Model file for the job. Use its own axes, mm. A direction names the side the tool comes from. Coordinates: 2 decimals unless noted, no trailing zeros. Order: outer loops, then holes, each group sorted by start corner. A loop starts at its lowest first (then second) coordinate and runs counter-clockwise, first axis right, second up.
from build123d import *

# Parameters (mm, degrees)
BOSS_EXTRUDE1_DEPTH      = 10
BOSS_EXTRUDE2_DEPTH      = 15
BOSS_EXTRUDE2_DEPTH_BACK = 25
SKETCH2_W                = 13.86324318
SKETCH2_H                = 2.640648634
SKETCH3_R                = 3.15
CUT_EXTRUDE1_DEPTH       = 2.65
BOSS_EXTRUDE3_DEPTH      = 10
SKETCH5_R                = 3.15
CUT_EXTRUDE2_DEPTH       = 10
BOSS_EXTRUDE4_DEPTH      = 15
BOSS_EXTRUDE4_DEPTH_BACK = 25
SKETCH7_W                = 13.86324318
SKETCH7_H                = 33.4262151
CUT_EXTRUDE3_DEPTH       = 15
SKETCH13_W               = 7.942289342
SKETCH13_H               = 13.358433402
SKETCH13_H_2             = 13.079806518
CUT_EXTRUDE4_DEPTH       = 35


with BuildPart() as part:
    # Sketch1 → Boss-Extrude1 (new body)
    with BuildSketch(Plane.XY):
        with BuildLine():
            Line((-102.490463188, 678.270987862), (-97.502783366, 678.270987862))
            ThreePointArc((-97.502783366, 678.270987862), (-96.402724844, 679.006023468), (-96.660835024, 680.30363097))
            Line((-96.660835024, 680.30363097), (-101.554583476, 685.197379422))
            ThreePointArc((-101.554583476, 685.197379422), (-102.523344038, 685.844684534), (-103.666075035, 686.071987862))
            Line((-103.666075035, 686.071987862), (-109.332102168, 686.071987862))
            ThreePointArc((-109.332102168, 686.071987862), (-110.474833165, 685.844684534), (-111.443593727, 685.197379422))
            Line((-111.443593727, 685.197379422), (-116.337342179, 680.30363097))
            ThreePointArc((-116.337342179, 680.30363097), (-116.595452359, 679.006023468), (-115.495393837, 678.270987862))
            Line((-115.495393837, 678.270987862), (-112.290288601, 678.270987862))
            Line((-112.290288601, 678.270987862), (-110.43275253, 678.270987862))
            Line((-110.43275253, 678.270987862), (-110.43275253, 674.001864678))
            Line((-110.43275253, 674.001864678), (-113.469742626, 674.001864678))
            Line((-113.469742626, 674.001864678), (-113.469742626, 640.576503739))
            Line((-113.469742626, 640.576503739), (-113.469742626, 637.935000944))
            Line((-113.469742626, 637.935000944), (-99.606499446, 637.935000944))
            Line((-99.606499446, 637.935000944), (-99.606499446, 674.001864678))
            Line((-99.606499446, 674.001864678), (-102.490463188, 674.001864678))
            Line((-102.490463188, 674.001864678), (-102.490463188, 678.270987862))
        make_face()
    extrude(amount=-BOSS_EXTRUDE1_DEPTH)

    # Sketch2 → Boss-Extrude2 (add, two sides: drawn at the far end of the back side and taken through both)
    with BuildSketch(Plane.XY.offset(-BOSS_EXTRUDE2_DEPTH_BACK)):
        with Locations((-106.538121036, 639.255325261)):
            Rectangle(SKETCH2_W, SKETCH2_H)
    extrude(amount=BOSS_EXTRUDE2_DEPTH + BOSS_EXTRUDE2_DEPTH_BACK)

    # Sketch3 → Cut-Extrude1 (cut)
    with BuildSketch(Plane(origin=(0, 640.575649578, 0), x_dir=(1, 0, 0), z_dir=(0, 1, 0))):
        with Locations(Location((-106.538121036, -7.5, 0), (0, 0, 270))):
            Circle(SKETCH3_R)
    extrude(amount=-CUT_EXTRUDE1_DEPTH, mode=Mode.SUBTRACT)

    # Sketch4 → Boss-Extrude3 (add)
    # profile 1 of 2: a face of its own
    with BuildSketch(Plane(origin=(0, 0, -10), x_dir=(-1, 0, 0), z_dir=(0, 0, -1))):
        Polygon((99.606499446, 637.935000944), (79.606499446, 637.935000944), (99.606499446, 674.001864678), align=None)
        Polygon((84.700453543, 640.935000944), (96.606499446, 662.405687703), (96.606499446, 640.935000944), align=None, mode=Mode.SUBTRACT)
    # profile 2 of 2: a face of its own
    with BuildSketch(Plane(origin=(0, 0, -10), x_dir=(-1, 0, 0), z_dir=(0, 0, -1))):
        Polygon((113.469742626, 637.935000944), (133.469742626, 637.935000944), (113.469742626, 674.001864678), align=None)
        Polygon((116.469742626, 662.405687703), (116.469742626, 640.935000944), (128.375788529, 640.935000944), align=None, mode=Mode.SUBTRACT)
    extrude(amount=-BOSS_EXTRUDE3_DEPTH)

    # Sketch5 → Cut-Extrude2 (cut)
    with BuildSketch(Plane(origin=(0, 640.575649578, 0), x_dir=(1, 0, 0), z_dir=(0, 1, 0))):
        with Locations(Location((-106.538121036, 17.5, 0), (0, 0, 270))):
            Circle(SKETCH5_R)
    extrude(amount=-CUT_EXTRUDE2_DEPTH, mode=Mode.SUBTRACT)

    # Sketch7 → Boss-Extrude4 (add, two sides: drawn at the far end of the back side and taken through both)
    with BuildSketch(Plane(origin=(0, 0, -10), x_dir=(-1, 0, 0), z_dir=(0, 0, -1)).offset(-BOSS_EXTRUDE4_DEPTH_BACK)):
        with Locations((106.538121036, 657.288757128)):
            Rectangle(SKETCH7_W, SKETCH7_H)
    extrude(amount=BOSS_EXTRUDE4_DEPTH + BOSS_EXTRUDE4_DEPTH_BACK)

    # Sketch10 → Cut-Extrude3 (cut)
    with BuildSketch(Plane(origin=(-99.606499446, 0, 0), x_dir=(0, 0, -1), z_dir=(1, 0, 0))):
        Polygon((25, 674.001864678), (10, 674.001864678), (25, 640.935000944), align=None)
        Polygon((-15, 640.935000944), (0, 674.001864678), (-15, 674.001864678), align=None)
    extrude(amount=-CUT_EXTRUDE3_DEPTH, mode=Mode.SUBTRACT)

    # Sketch13 → Cut-Extrude4 (cut)
    with BuildSketch(Plane(origin=(0, 674.001864678, 0), x_dir=(1, 0, 0), z_dir=(0, 1, 0))):
        with Locations((-106.461607859, -6.679216701)):
            Rectangle(SKETCH13_W, SKETCH13_H)
        with Locations((-106.461607859, 16.539903259)):
            Rectangle(SKETCH13_W, SKETCH13_H_2)
    extrude(amount=-CUT_EXTRUDE4_DEPTH, mode=Mode.SUBTRACT)


solid = part.part
Q1. Cut at A-A, the plane z = -5. List the corners of the cut face in (x, y) (1 decimal).
Established:
outline: (-133.5, 637.9) - (-79.6, 637.9) - (-99.6, 674) - (-102.5, 674) - (-102.5, 678.3) - (-97.5, 678.3) arc R1.2 ccw to (-96.7, 680.3) - (-101.6, 685.2) arc R3 ccw to (-103.7, 686.1) - (-109.3, 686.1) arc R3 ccw to (-111.4, 685.2) - (-116.3, 680.3) arc R1.2 ccw to (-115.5, 678.3) - (-110.4, 678.3) - (-110.4, 674) - (-113.5, 674) - close; hole (-128.4, 640.9) - (-116.5, 640.9) - (-116.5, 662.4) - close; hole (-96.6, 640.9) - (-84.7, 640.9) - (-96.6, 662.4) - close
Q2. Cut at B-B, the plane x = -127.5. List the corners of the cut face in (y, z) (1 decimal), plus the area to 3 significant figures.
Established:
outline: (637.9, -10) - (640.9, -10) - (640.9, 0) - (637.9, 0) - close; (642.5, -10) - (648.7, -10) - (648.7, 0) - (642.5, 0) - close
area: 91.9 mm2
Q3. Cut at C-C, the plane y = 649.5. List the corners of the cut face in (x, z).
Established:
outline: (-127.06, -10) - (-123.63, -10) - (-123.63, 0) - (-127.06, 0) - close; (-116.47, -10) - (-113.47, -10) - (-113.47, -21.11) - (-110.43, -21.11) - (-110.43, -10) - (-102.49, -10) - (-102.49, -21.11) - (-99.61, -21.11) - (-99.61, -10) - (-96.61, -10) - (-96.61, 0) - (-99.61, 0) - (-99.61, 11.11) - (-102.49, 11.11) - (-102.49, 0) - (-110.43, 0) - (-110.43, 11.11) - (-113.47, 11.11) - (-113.47, 0) - (-116.47, 0) - close; (-89.45, -10) - (-86.02, -10) - (-86.02, 0) - (-89.45, 0) - close
Q4. Cut at D-D, the plane x = -104.5. List the corners of the cut face in (y, z) (3 decimals), plus the area to 3 significant figures.
Established:
outline: (637.935, -25) - (640.935, -25) - (645.168, -23.08) - (639.002, -23.08) - (639.002, -19.902) - (637.935, -19.902) - close; (637.935, -15.098) - (639.002, -15.098) - (639.002, -10) - (686.072, -10) - (686.072, 0) - (639.002, 0) - (639.002, 5.098) - (637.935, 5.098) - close; (637.935, 9.902) - (639.002, 9.902) - (639.002, 13.358) - (644.554, 13.358) - (640.935, 15) - (637.935, 15) - close
area: 517 mm2
Q5. Which spindle directions (+Z, -Z, +X, -X, +Y, -Y) get a long thin tool onto all of the face, cutting with end or side? Do faces 4 (the face through (-100, 678.271, -5)), 5 (the face through (-122, 640.935, -5)), 6 (the face through (-102.49, 653, 5)), 7 (the face through (-110.433, 676, -5)). Say none if no direction does.
Established:
face 4: +Z, -Z, +X
face 5: +Z, -Z
face 6: +Y
face 7: +Z, -Z, -X
Q6. Probe line 1 (X direction, y = 638.55, z = -17.5); line 2 (X direction, y = 659, z = 1); line 3 (X direction, y = 676, z = -8). List the from-to ranges inside material, lowest first.
Established:
line 1: x = -113.47 to -109.69, -103.39 to -99.61
line 2: x = -113.47 to -110.43, -102.49 to -99.61
line 3: x = -110.43 to -102.49
Q7. Mould opens along X. For faces 1 (the face through (-97, 651, -10)), 2 (the face through (-110.46, 685.85, -4.93)), 3 (the face through (-91, 640.935, -5)) say: pulls with the +X half, pulls with the -X half, needs draft (parallel to the pull), parting line crosses it, or undercut.
Established:
face 1: needs draft
face 2: pulls with the -X half
face 3: undercut
Q8. Drop flat-ended pins along their axis: P1, Ø10, axis at x = -121.5, y = 652, coming from the +Z side; P2, Ø10.5, axis at y = 648, z = 3.5, coming from the +X side; P3, Ø2.5, axis at x = -111.5, z = -6, coming from the +Y side. Give the stop position or say it passes through.
Established:
P1: stops at z = 0
P2: stops at x = -83.02
P3: stops at y = 685.93
